Autodesk Inventor part; units mm, degrees
ref_plane "YZ Plane" through (0, 0, 0) normal (1, 0, 0) x (0, 1, 0)
ref_plane "XZ Plane" through (0, 0, 0) normal (0, 1, 0) x (-1, 0, 0)
ref_plane "XY Plane" through (0, 0, 0) normal (0, 0, 1) x (1, 0, 0)
sketch "Sketch1" plane through (0, 0, 0) normal (0, 0, 1) x (1, 0, 0)
  circle A0 centre (0, 0) radius 47.5
  circle A1 centre (0, 0) radius 52.5
  circle A2 centre (0, 50.35) radius 1.5
  circle A3 centre (-43.6044, 25.175) radius 1.5
  circle A4 centre (-43.6044, -25.175) radius 1.5
  circle A5 centre (0, -50.35) radius 1.5
  circle A6 centre (43.6044, -25.175) radius 1.5
  circle A7 centre (43.6044, 25.175) radius 1.5
  dimension "d0" = 95
  dimension "d1" = 105
  dimension "d2" = 3
  dimension "d5" = 360
  dimension "d9" = 1.35
extrude "Extrusion1" add sketch "Sketch1" along normal blind 1.5
properties part number "bead lock" material "PCTG 20%"
The model under review builds one solid part; all positions refer to its coordinate system, in mm. Coordinates: 2 decimals unless noted, no trailing zeros. Write each loop counter-clockwise with the first axis right and the second up, starting at its lowest first coordinate (ties: lowest second). Pieces come first, ordered by that corner, then holes. Notation, with made-up numbers: (59, 23) -> (63, 23) arc R22 cw to (63, 34) -> close; hole circle Ø4 at (41, -19). An arc over 180 degrees is marked (long way). Answer in a Markdown table with one row per item.
1. We need section A-A, the plane x = 0. State the section outline as (y, z) points.
Answers below:
| item | result |
|---|---|
| outline | (-52.5, 0) -> (-51.85, 0) -> (-51.85, 1.5) -> (-52.5, 1.5) -> close; (-48.85, 0) -> (-47.5, 0) -> (-47.5, 1.5) -> (-48.85, 1.5) -> close; (47.5, 0) -> (48.85, 0) -> (48.85, 1.5) -> (47.5, 1.5) -> close; (51.85, 0) -> (52.5, 0) -> (52.5, 1.5) -> (51.85, 1.5) -> close |
2. Wall thickness on probe 1 along Y at (x, z) = (0, 0.5); probe 2 along X at (y, z) = (-24, 1.25); probe 3 along Y at (x, z) = (23, 0.45): over which ranges is each line inside the solid? List them lowest first. Write a range as [from, to].
Answers below:
| item | result |
|---|---|
| probe 1 | y = [-52.5, -51.85], [-48.85, -47.5], [47.5, 48.85], [51.85, 52.5] |
| probe 2 | x = [-46.69, -44.54], [-42.67, -40.99], [40.99, 42.67], [44.54, 46.69] |
| probe 3 | y = [-47.19, -41.56], [41.56, 47.19] |
3. We need section D-D, the plane z = 0.65. State the section outline as (x, y) points (3 decimals), and give its area (3 significant figures).
Answers below:
| item | result |
|---|---|
| outline | circle Ø105 at (0, 0); hole circle Ø95 at (0, 0); hole circle Ø3 at (-43.604, -25.175); hole circle Ø3 at (-43.604, 25.175); hole circle Ø3 at (0, -50.35); hole circle Ø3 at (0, 50.35); hole circle Ø3 at (43.604, -25.175); hole circle Ø3 at (43.604, 25.175) |
| area | 1,530 mm^2 |
4. We need section C-C, the plane x = -35. State the section outline as (y, z) points, and give its area (3 significant figures).
Answers below:
| item | result |
|---|---|
| outline | (-39.13, 0) -> (-32.11, 0) -> (-32.11, 1.5) -> (-39.13, 1.5) -> close; (32.11, 0) -> (39.13, 0) -> (39.13, 1.5) -> (32.11, 1.5) -> close |
| area | 21.1 mm^2 |
5. We need section B-B, the plane y = 39. State the section outline as (x, z) points.
Answers below:
| item | result |
|---|---|
| outline | (-35.15, 0) -> (-27.12, 0) -> (-27.12, 1.5) -> (-35.15, 1.5) -> close; (27.12, 0) -> (35.15, 0) -> (35.15, 1.5) -> (27.12, 1.5) -> close |
6. Draft analysis for pull direction Y (two halves, no side actions). For faces 1 (the cylindrical face through (-0.195, 48.863, 0.74)), 2 (the cylindrical face through (-44.71, 24.16, 0.74)), 3 (the flat face through (-27.5, 39.1, 1.5)), 4 (the cylindrical face through (50.076, -15.77, 0.74)), state which applies: +Y half, -Y half, draft (parallel to the pull), parting line (faces both ways), or undercut.
Answers below:
| item | result |
|---|---|
| face 1 | undercut |
| face 2 | undercut |
| face 3 | draft |
| face 4 | parting line |
